```python
from build123d import *

# Parameters (mm, degrees)
CUT_EXTRUDE1_DEPTH  = 16
SKETCH4_R           = 1
BOSS_EXTRUDE1_DEPTH = 0.75
CIRPATTERN1_COUNT   = 4


with BuildPart() as part:
    # Sketch2 → Revolve1 (revolve)
    with BuildSketch(Plane.XY, mode=Mode.PRIVATE) as revolve1_sk:
        with BuildLine():
            Line((0, 2.5), (0, -2.5))
            Line((0, -2.5), (10, -2.5))
            Line((10, -2.5), (10, -1.969615506))
            ThreePointArc((10, -1.969615506), (8.347296355, 0), (10, 1.969615506))
            Line((10, 1.969615506), (10, 2.5))
            Line((10, 2.5), (0, 2.5))
        make_face()
    revolve(revolve1_sk.sketch.rotate(Axis((0, 0, 0), (0, 1, 0)), 90), axis=Axis((0, 0, 0), (0, 1, 0)))

    # Sketch3 → Cut-Extrude1 (cut, through all)
    with BuildSketch(Plane(origin=(0, 2.5, 0), x_dir=(1, 0, 0), z_dir=(0, 1, 0))):
        with BuildLine():
            Line((-1.658312395, 2.5), (1.658312395, 2.5))
            ThreePointArc((1.658312395, 2.5), (0, -3), (-1.658312395, 2.5))
        make_face()
    extrude(amount=-CUT_EXTRUDE1_DEPTH, mode=Mode.SUBTRACT)

    # Sketch4 → Boss-Extrude1 (add, symmetric)
    with BuildSketch(Plane(origin=(0, 0, 0), x_dir=(1, 0, 0), z_dir=(0, 1, 0))):
        with BuildLine():
            Line((5.347296355, 2), (10.347296355, 2))
            ThreePointArc((10.347296355, 2), (12.347296355, 0), (10.347296355, -2))
            Line((10.347296355, -2), (5.347296355, -2))
            Line((5.347296355, -2), (5.347296355, 2))
        make_face()
        with Locations(Location((10.347296355, 0, 0), (0, 0, 270))):
            Circle(SKETCH4_R, mode=Mode.SUBTRACT)
    boss_extrude1 = extrude(amount=BOSS_EXTRUDE1_DEPTH, both=True)

    # CirPattern1: Boss-Extrude1 ×4 about axis
    cirpattern1_axis = Axis((0, 0, 0), (0, 1, 0))
    for i in range(1, CIRPATTERN1_COUNT):
        add(boss_extrude1.rotate(cirpattern1_axis, i * 360 / CIRPATTERN1_COUNT))


solid = part.part
```
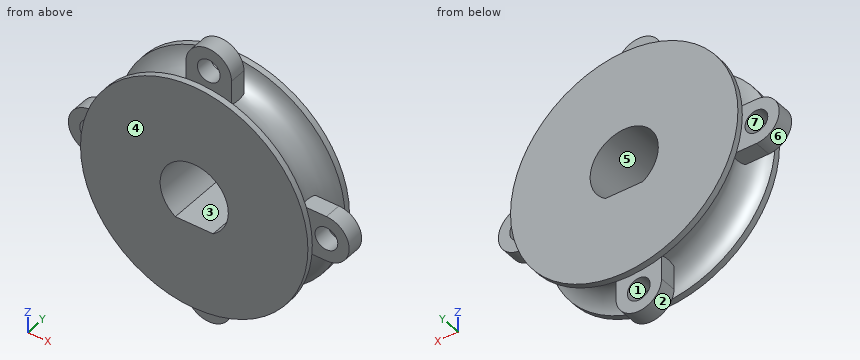
Here's how the part is built. I have some questions about the finished solid (model axes, mm). Face numbers are marked on the shaded views. A direction names the side the tool comes from. Coordinates: 2 decimals unless noted, no trailing zeros. Order: outer loops, then holes, each group sorted by start corner. A loop starts at its lowest first (then second) coordinate and runs counter-clockwise, first axis right, second up. Notation, with made-up numbers: (-17, 44.25) - (6, 44.25) arc R25 cw to (6, 81.25) - close; hole circle Ø11 at (63.5, 82.5). An arc over 180 degrees is marked (long way). One line per question, with ' | ' between items. Start each with the question number.
1. Please list where these lines run through material, in increasing order: line 1 along X through (y, z) = (0.4, 0); line 2 along Z through (x, y) = (0, -0.2); line 3 along Z through (x, y) = (-9.5, 0.05). Write a range as [from, to].
2. If we section it at A-A (x = 0): Write out the boundary of the cut face in (y, z).
3. Which directions (+Z, -Z, +X, -X, +Y, -Y) give clear straight access to the entire face, cutting with the end or side of a thin tool? Please do the marked faces 1, 2 and 3.
4. If we mould it in two halves opening along Z, with no side actions, what happens to the marked faces 4, 5, 6 and 7? For each: released by +Z, released by -Z, zero draft, split by the parting line, or undercut.
5. If we section it at C-C (x = 9): Give the number of separate pieces and of enclosed holes in the cut face, and give its area (3 significant figures).
6. I'm going to push flat-ended pins straight in: pin 1 Ø0.8 at (y, z) = (0, -9.5) entering from +X; pin 2 Ø2.5 at (x, z) = (0, 10.35) entering from -Y; pin 3 Ø0.5 at (x, y) = (9, 0) entering from -Z; pin 4 Ø1.7 at (y, z) = (0, 9) entering from -X. Where does each tip first touch, or does it pass through?
7. If we section it at B-B (z = 0): Write out the boundary of the cut face in (x, y), and give its area (3 significant figures).
Model answer:
1) line 1: x = [-12.35, -11.35], [-9.35, -3], [3, 9.35], [11.35, 12.35] | line 2: z = [-12.35, -11.35], [-9.35, -2.5], [3, 9.35], [11.35, 12.35] | line 3: z = [-2, -0.53], [0.53, 2]
2) outline: (-2.5, -10) - (-1.97, -10) arc R2 cw to (-0.75, -8.49) - (-0.75, -9.35) - (0.75, -9.35) - (0.75, -8.49) arc R2 cw to (1.97, -10) - (2.5, -10) - (2.5, -2.5) - (-2.5, -2.5) - close; (-2.5, 3) - (2.5, 3) - (2.5, 10) - (1.97, 10) arc R2 cw to (0.75, 8.49) - (0.75, 9.35) - (-0.75, 9.35) - (-0.75, 8.49) arc R2 cw to (-1.97, 10) - (-2.5, 10) - close; (-0.75, -12.35) - (0.75, -12.35) - (0.75, -11.35) - (-0.75, -11.35) - close; (-0.75, 11.35) - (0.75, 11.35) - (0.75, 12.35) - (-0.75, 12.35) - close
3) face 1: none | face 2: -Z, +Y, -Y | face 3: +Y, -Y
4) face 4: zero draft | face 5: undercut | face 6: split by the parting line | face 7: undercut
5) separate pieces: 3 | enclosed holes: 0 | area: 20.1 mm²
6) pin 1: stops at x = 2 | pin 2: stops at y = -2.5 | pin 3: stops at z = -2 | pin 4: stops at x = -2
7) outline: (-12.35, -0.75) - (-11.35, -0.75) - (-11.35, 0.75) - (-12.35, 0.75) - close; (-10, -2.5) - (-3, -2.5) - (-3, 2.5) - (-10, 2.5) - (-10, 1.97) arc R2 cw to (-8.49, 0.75) - (-9.35, 0.75) - (-9.35, -0.75) - (-8.49, -0.75) arc R2 cw to (-10, -1.97) - close; (3, -2.5) - (10, -2.5) - (10, -1.97) arc R2 cw to (8.49, -0.75) - (9.35, -0.75) - (9.35, 0.75) - (8.49, 0.75) arc R2 cw to (10, 1.97) - (10, 2.5) - (3, 2.5) - close; (11.35, -0.75) - (12.35, -0.75) - (12.35, 0.75) - (11.35, 0.75) - close | area: 66.1 mm²
